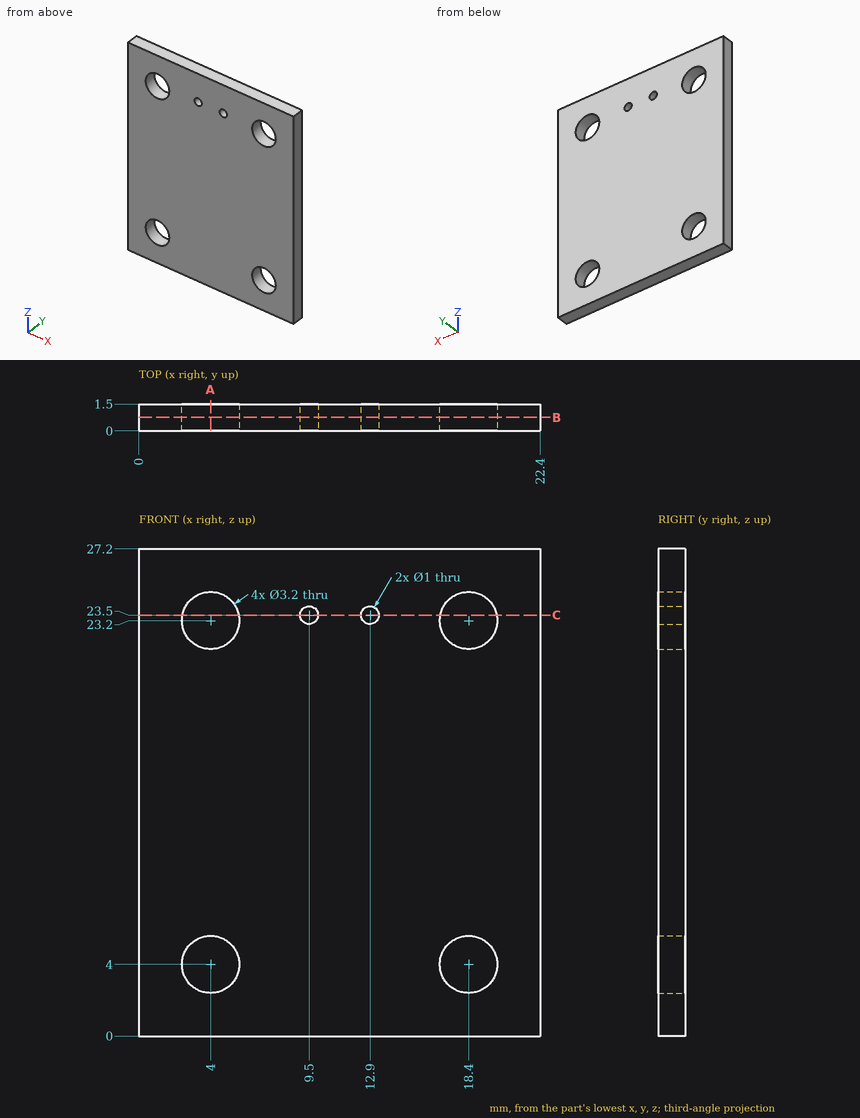
Study the drawing (mm; zero at the part's minimum x, y, z) and answer. Coordinates: 2 decimals unless noted, no trailing zeros. Write each loop counter-clockwise with the first axis right and the second up, starting at its lowest first coordinate (ties: lowest second). Pieces come first, ordered by that corner, then holes.
Q1. This flat-tipped pin is pushed along its axis until it touches: pin 1 Ø3.5 at (x, z) = (18.4, 4) entering from +Y. Where does it stop, or does it pass through?
Q2. A cutting plane is placed at A-A, the plane x = 4. Give the vertices of the cut face in (y, z).
Q3. A cutting plane is placed at C-C, the plane z = 23.5. Give the vertices of the cut face in (x, y).
Q4. Find the intervals of material crossed by line 1 (Z direction, x = 18.4, y = 1.05); line 2 (Z direction, x = 19.5, y = 0.3); line 3 (Z direction, x = 9.5, y = 1.15), in increasing order.
Q5. A cutting plane is placed at B-B, the plane y = 0.75. Give the vertices of the cut face in (x, z), then the cut area to 3 significant figures.
Findings below:
1. pin 1: stops at y = 1.5
2. outline: (0, 0) - (1.5, 0) - (1.5, 2.4) - (0, 2.4) - close; (0, 5.6) - (1.5, 5.6) - (1.5, 21.6) - (0, 21.6) - close; (0, 24.8) - (1.5, 24.8) - (1.5, 27.2) - (0, 27.2) - close
3. outline: (0, 0) - (2.43, 0) - (2.43, 1.5) - (0, 1.5) - close; (5.57, 0) - (9, 0) - (9, 1.5) - (5.57, 1.5) - close; (10, 0) - (12.4, 0) - (12.4, 1.5) - (10, 1.5) - close; (13.4, 0) - (16.83, 0) - (16.83, 1.5) - (13.4, 1.5) - close; (19.97, 0) - (22.4, 0) - (22.4, 1.5) - (19.97, 1.5) - close
4. line 1: z = 0 to 2.4, 5.6 to 21.6, 24.8 to 27.2
4. line 2: z = 0 to 2.84, 5.16 to 22.04, 24.36 to 27.2
4. line 3: z = 0 to 23, 24 to 27.2
5. outline: (0, 0) - (22.4, 0) - (22.4, 27.2) - (0, 27.2) - close; hole circle Ø3.2 at (4, 4); hole circle Ø3.2 at (4, 23.2); hole circle Ø1 at (9.5, 23.5); hole circle Ø1 at (12.9, 23.5); hole circle Ø3.2 at (18.4, 4); hole circle Ø3.2 at (18.4, 23.2)
5. area: 576 mm2
